from build123d import *

# Parameters (mm, degrees)
F0_W        = 12
F0_H        = 15
F1_DEPTH    = 5
F2_W        = 12
F2_H        = 6.5
F3_DEPTH    = 33
F4_W        = 6.5
F4_H        = 33
F5_DEPTH    = 25
F6_T1_DEPTH = 12
F7_R        = 3.25
F8_DEPTH    = 25
F9_W        = 6.5
F9_H        = 0.5
F10_DEPTH   = 25
F11_R       = 5


# Not quite as in the source:
# - a fillet or chamfer that OpenCascade refuses, or shapes differently, is made with other operations: its cross-section is extruded or revolved along the edge and cut away or added


with BuildPart() as f1:
    # F0 (on Top) → F1 (new body)
    with BuildSketch(Plane.XY):
        Rectangle(F0_W, F0_H)
    extrude(amount=F1_DEPTH)

    # F2 (on face) → F3 (join)
    with BuildSketch(Plane.XY.offset(5)):
        Rectangle(F2_W, F2_H)
    extrude(amount=F3_DEPTH)

    # F4 (on face) → F5 (join)
    with BuildSketch(Plane(origin=(-6, 0, 0), x_dir=(0, -1, 0), z_dir=(-1, 0, 0))):
        with Locations((0, 21.5)):
            Rectangle(F4_W, F4_H)
    extrude(amount=F5_DEPTH)

    # F6: fillet of radius 5 on 2 edges, made by hand

    # F6_s2 → F6_t1 (join)
    with BuildSketch(Plane.YZ.offset(-6)):
        with BuildLine():
            ThreePointArc((-3.25, 9.9434299833), (-4.458562278, 6.6838287807), (-7.5, 5))
            Line((-7.5, 5), (-3.25, 5))
            Line((-3.25, 5), (-3.25, 9.9434299833))
        make_face()
        with BuildLine():
            ThreePointArc((7.5, 5), (4.458562278, 6.6838287807), (3.25, 9.9434299833))
            Line((3.25, 9.9434299833), (3.25, 5))
            Line((3.25, 5), (7.5, 5))
        make_face()
    extrude(amount=F6_T1_DEPTH)

    # F7 (on face) → F8 (cut)
    with BuildSketch(Plane.XZ.offset(3.25)):
        with Locations((-18.7, 22)):
            Circle(F7_R)
    extrude(amount=-F8_DEPTH, mode=Mode.SUBTRACT)

    # F9 (on face) → F10 (cut)
    with BuildSketch(Plane(origin=(-31, 0, 0), x_dir=(0, -1, 0), z_dir=(-1, 0, 0))):
        with Locations((0, 5.25)):
            Rectangle(F9_W, F9_H)
    extrude(amount=-F10_DEPTH, mode=Mode.SUBTRACT)

    # F11
    f11_edges = [f1.edges().sort_by_distance(p)[0] for p in [
        (-31, 0, 38),
    ]]
    fillet(f11_edges, radius=F11_R)


solid = f1.part
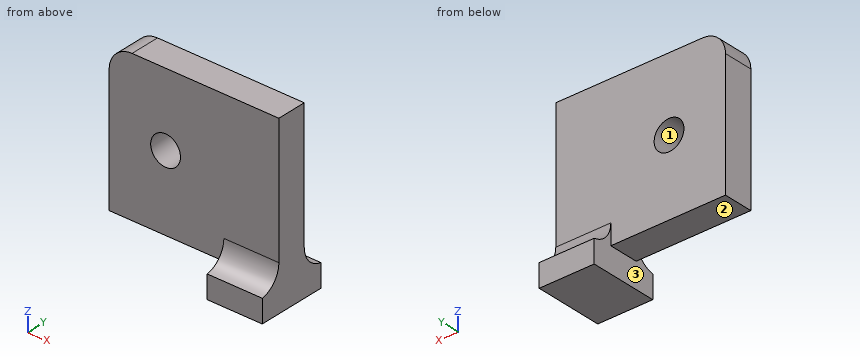
Build history of the part. All positions in model axes, mm. Face numbers are marked on the shaded views. Coordinates: 2 decimals unless noted, no trailing zeros. Write each loop counter-clockwise with the first axis right and the second up, starting at its lowest first coordinate (ties: lowest second). Pieces come first, ordered by that corner, then holes.
(1) Drill centre lines: line 1 (Z direction, x = -18.7, y = 0.75); line 2 (Y direction, x = -7, z = 10); line 3 (Z direction, x = -10.5, y = 1.5). Where is each one in solid material? Low to high.
(2) Mould opens along Z. For the marked faces 1, 2 and 3 say: pulls with the +Z half, pulls with the -Z half, needs draft (parallel to the pull), parting line crosses it, or undercut.
(3) Cut at B-B on y = 1.5. List the corners of the cut face in (x, z), and give its area (3 significant figures).
(4) Pin check, flat tips, straight feed: pin 1 Ø5 at (x, z) = (-27, 25.5) entering from -Y; pin 2 Ø1 at (x, y) = (-2.5, -5.5) entering from +Z; pin 3 Ø16 at (x, z) = (-12.5, 17.5) entering from +Y. Stop position of each tip, or through.
(5) Cut at C-C on z = 22. List the corners of the cut face in (x, y).
(6) Cut at D-D on z = 8. List the corners of the cut face in (x, y), and give its area (3 significant figures).
(7) Cut at A-A on x = -18.7. List the corners of the cut face in (y, z).
Working result:
1. line 1: z = 5.5 to 18.75, 25.25 to 38
1. line 2: y = -3.25 to 3.25
1. line 3: z = 5.5 to 38
2. face 1: undercut
2. face 2: pulls with the -Z half
2. face 3: needs draft
3. outline: (-31, 5.5) - (-6, 5.5) - (-6, 0) - (6, 0) - (6, 38) - (-26, 38) arc R5 ccw to (-31, 33) - close; hole circle Ø6.5 at (-18.7, 22)
3. area: 1,230 mm2
4. pin 1: stops at y = -3.25
4. pin 2: stops at z = 6.14
4. pin 3: stops at y = 3.25
5. outline: (-31, -3.25) - (-21.95, -3.25) - (-21.95, 3.25) - (-31, 3.25) - close; (-15.45, -3.25) - (6, -3.25) - (6, 3.25) - (-15.45, 3.25) - close
6. outline: (-31, -3.25) - (-6, -3.25) - (-6, -3.64) - (6, -3.64) - (6, 3.64) - (-6, 3.64) - (-6, 3.25) - (-31, 3.25) - close
6. area: 250 mm2
7. outline: (-3.25, 5.5) - (3.25, 5.5) - (3.25, 18.75) - (-3.25, 18.75) - close; (-3.25, 25.25) - (3.25, 25.25) - (3.25, 38) - (-3.25, 38) - close
